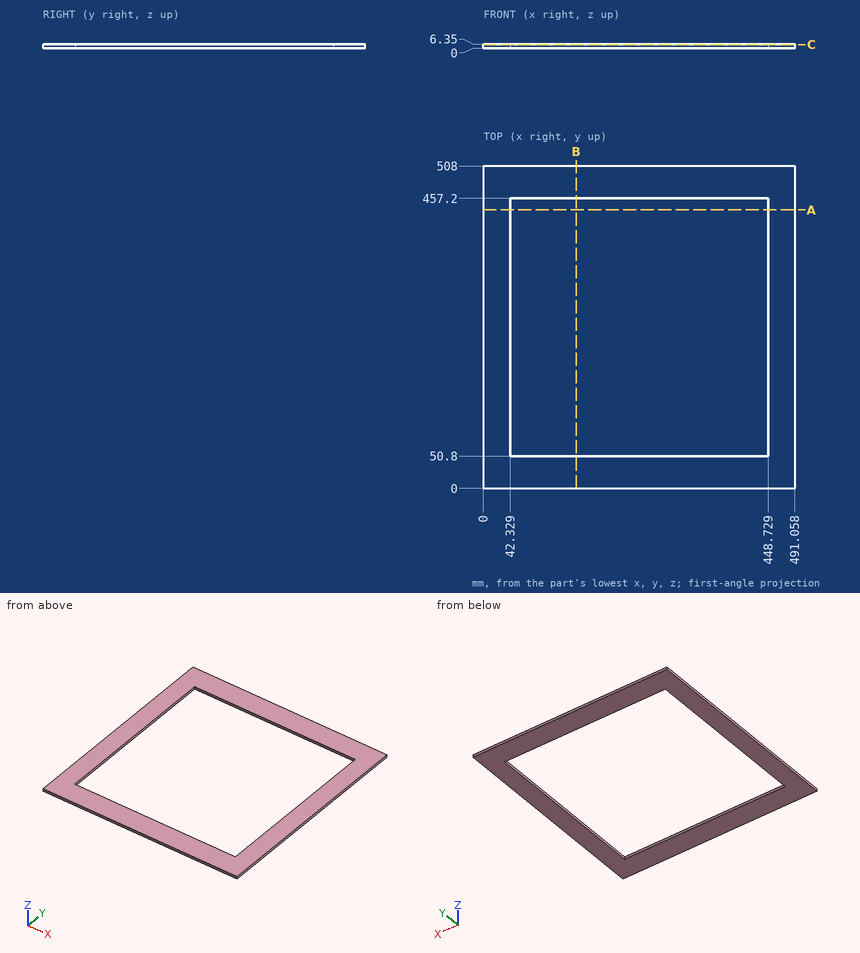
Design review of the part shown in the three views and the two pictorial views. Dimensions are in mm from the part's minimum x, y and z. Give positions to 0.01 mm unless a question says otherwise; leave off trailing zeros. Write each loop counter-clockwise with the first axis right and the second up, starting at its lowest first coordinate (ties: lowest second). Pieces come first, ordered by that corner, then holes. Notation, with made-up numbers: M 47,83 L 82,83 A30 ccw 82,109 Z; hole C 84.25,89 d6. An arc over 180 degrees is marked long. One line per item, written item: value.
1) Take a section at A-A, the plane y = 439. Write out the cut boundary in (x, z), then the cut area to 3 significant figures.
Results are:
outline: M 0,0 L 42.33,0 L 42.33,6.35 L 0,6.35 Z; M 448.73,0 L 491.06,0 L 491.06,6.35 L 448.73,6.35 Z
area: 538 mm²
2) Take a section at B-B, the plane x = 146. Write out the cut boundary in (y, z).
Results are:
outline: M 0,0 L 50.8,0 L 50.8,6.35 L 0,6.35 Z; M 457.2,0 L 508,0 L 508,6.35 L 457.2,6.35 Z
3) For line 1 (X direction, y = 185.5, z = 1); line 2 (Y direction, x = 440.5, z = 5.25), list the stretches that pass through material, from the lowest coordinate up. Write a range as from..to.
Results are:
line 1: x = 0..42.33, 448.73..491.06
line 2: y = 0..50.8, 457.2..508
4) Take a section at C-C, the plane z = 5.25. Write out the cut boundary in (x, y).
Results are:
outline: M 0,0 L 491.06,0 L 491.06,508 L 0,508 Z; hole M 42.33,50.8 L 448.73,50.8 L 448.73,457.2 L 42.33,457.2 Z
